Here's how the part is built. I have some questions about the finished solid (model axes, mm). A direction names the side the tool comes from. Give positions to 0.01 mm unless a question says otherwise; leave off trailing zeros. Order: outer loops, then holes, each group sorted by start corner. A loop starts at its lowest first (then second) coordinate and runs counter-clockwise, first axis right, second up. Notation, with made-up numbers: M 8.25,-13 L 30.25,-13 A23 cw 30.25,24 Z; hole C -10,13 d9. An arc over 180 degrees is marked long. One line per item, written item: value. Start each with the question number.
from build123d import *

# Parameters (mm, degrees)
SKETCH1_W           = 24.25
SKETCH1_H           = 35.375
SKETCH1_R           = 1
SKETCH1_W_2         = 16.25
SKETCH1_W_3         = 11.5
SKETCH1_R_2         = 2.875
BOSS_EXTRUDE1_DEPTH = 65
CUT_EXTRUDE1_START  = 65
SKETCH1_3_R         = 1
CUT_EXTRUDE1_DEPTH  = 15
SKETCH1_4_W         = 24.25
SKETCH1_4_H         = 35.375
SKETCH1_4_R         = 1
BOSS_EXTRUDE2_DEPTH = 44
SKETCH1_5_R         = 2.875
BOSS_EXTRUDE3_DEPTH = 9
BOSS_EXTRUDE3_TAPER = 3


with BuildPart() as part:
    # Sketch1 → Boss-Extrude1 (new body)
    with BuildSketch(Plane(origin=(0, 0, 0), x_dir=(1, 0, 0), z_dir=(0, 1, 0))):
        with Locations((-28.375, 17.6875)):
            Rectangle(SKETCH1_W, SKETCH1_H)
        with Locations((-25.25, 25.375)):
            Circle(SKETCH1_R, mode=Mode.SUBTRACT)
        with Locations((-8.125, 17.6875)):
            Rectangle(SKETCH1_W_2, SKETCH1_H)
        with Locations((-3.75, 25.375)):
            Circle(SKETCH1_R, mode=Mode.SUBTRACT)
        with Locations((5.75, 17.6875)):
            Rectangle(SKETCH1_W_3, SKETCH1_H)
        Polygon((11.5, 0), (0, 0), (-16.25, 0), (-40.5, 0), (-40.5, -16.25), (11.5, -16.25), align=None)
        with Locations((-30.5, -8.125)):
            Circle(SKETCH1_R_2, mode=Mode.SUBTRACT)
        with Locations((-25.25, -8.125)):
            Circle(SKETCH1_R, mode=Mode.SUBTRACT)
        with Locations((-3.75, -8.125)):
            Circle(SKETCH1_R, mode=Mode.SUBTRACT)
        with Locations((1.5, -8.125)):
            Circle(SKETCH1_R_2, mode=Mode.SUBTRACT)
        with Locations((-30.5, -8.125)):
            Circle(SKETCH1_R_2)
        with Locations((1.5, -8.125)):
            Circle(SKETCH1_R_2)
        with Locations((-3.75, -8.125)):
            Circle(SKETCH1_R)
        with Locations((-3.75, 25.375)):
            Circle(SKETCH1_R)
        with Locations((-25.25, 25.375)):
            Circle(SKETCH1_R)
        with Locations((-25.25, -8.125)):
            Circle(SKETCH1_R)
    extrude(amount=BOSS_EXTRUDE1_DEPTH)

    # Sketch1<3> → Cut-Extrude1 (cut)
    with BuildSketch(Plane(origin=(0, 0, 0), x_dir=(1, 0, 0), z_dir=(0, 1, 0)).offset(CUT_EXTRUDE1_START)):
        with Locations((-3.75, -8.125)):
            Circle(SKETCH1_3_R)
        with Locations((-25.25, -8.125)):
            Circle(SKETCH1_3_R)
        with Locations((-3.75, 25.375)):
            Circle(SKETCH1_3_R)
        with Locations((-25.25, 25.375)):
            Circle(SKETCH1_3_R)
    extrude(amount=-CUT_EXTRUDE1_DEPTH, mode=Mode.SUBTRACT)

    # Sketch1<4> → Boss-Extrude2 (add)
    with BuildSketch(Plane(origin=(0, 0, 0), x_dir=(1, 0, 0), z_dir=(0, 1, 0))):
        with Locations((-28.375, 17.6875)):
            Rectangle(SKETCH1_4_W, SKETCH1_4_H)
        with Locations((-25.25, 25.375)):
            Circle(SKETCH1_4_R, mode=Mode.SUBTRACT)
        with Locations((-25.25, 25.375)):
            Circle(SKETCH1_4_R)
    extrude(amount=-BOSS_EXTRUDE2_DEPTH)

    # Sketch1<5> → Boss-Extrude3 (add)
    with BuildSketch(Plane(origin=(0, 0, 0), x_dir=(1, 0, 0), z_dir=(0, 1, 0))):
        with Locations((1.5, -8.125)):
            Circle(SKETCH1_5_R)
        with Locations((-30.5, -8.125)):
            Circle(SKETCH1_5_R)
    extrude(amount=-BOSS_EXTRUDE3_DEPTH, taper=BOSS_EXTRUDE3_TAPER)


solid = part.part
Item 1: Will these pins go through, and if not, where does the flat tip stop? P1, Ø19.5, axis at x = -29.5, y = -31, coming from the +Z side; P2, Ø12, axis at x = 4, z = 1, coming from the -Y side; P3, Ø2.5, axis at x = -3.75, z = 8.125, coming from the -Y side.
Item 2: Please list where these lines run through material, in increasing order: probe 1 along Z at (x, y) = (-25.25, 59) (3 decimals); probe 2 along Y at (x, z) = (-14, -6); probe 3 along X at (y, z) = (-22.5, -22.5). Write a range as [from, to].
Item 3: We'd pull the mould along X, two halves only. Please class faces 1 (the face through (11.5, 32, -9)), 2 (the face through (0.93, -4.56, 10.7)), 3 (the face through (-21, 23, -35.375)), 4 (the face through (-25, 50, -25)): +X half, -X half, draft (parallel to the pull), parting line (faces both ways), or undercut.
Item 4: For faces 5 (the face through (-3.88, 57.605, 7.134)), 6 (the face through (-40.5, 11, -15)), which set-ups out of +Z, -Z, +X, -X, +Y, -Y let a thin tool reach every point of the face, with its end or its side?
Item 5: I want a section at B-B on y = -21. Write out the boundary of the cut face in (x, z) (3 decimals), plus the area to 3 significant figures.
Item 6: I want a section at A-A on z = -18. Write out the boundary of the cut face in (x, y), plus the area to 3 significant figures.
Item 7: I want a section at C-C on x = 6.5. Write out the boundary of the cut face in (y, z) (3 decimals).
Answer below:
1. P1: stops at z = 0
1. P2: stops at y = -9
1. P3: stops at y = 0
2. probe 1: z = [-35.375, -26.375], [-24.375, 7.125], [9.125, 16.25]
2. probe 2: y = [0, 65]
2. probe 3: x = [-40.5, -16.25]
3. face 1: +X half
3. face 2: undercut
3. face 3: draft
3. face 4: undercut
4. face 5: +Y
4. face 6: +Z, -Z, -X, +Y, -Y
5. outline: M -40.5,-35.375 L -16.25,-35.375 L -16.25,0 L -40.5,0 Z
5. area: 858 mm²
6. outline: M -40.5,-44 L -16.25,-44 L -16.25,0 L 11.5,0 L 11.5,65 L -40.5,65 Z
6. area: 4,450 mm²
7. outline: M 0,-35.375 L 65,-35.375 L 65,16.25 L 0,16.25 Z
